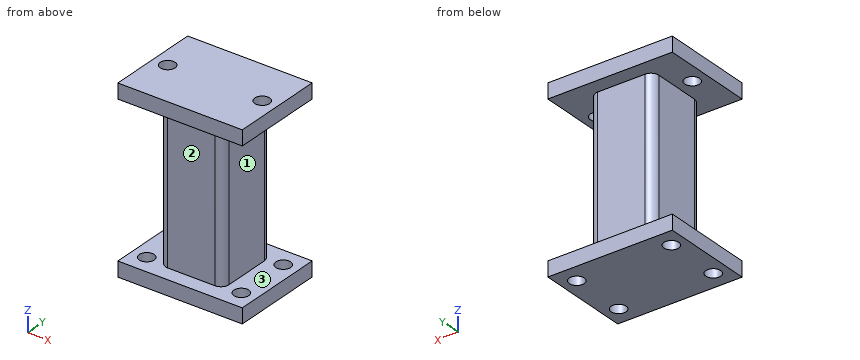
```python
from build123d import *

# Parameters (mm, degrees)
F0_W     = 100
F0_H     = 75
F1_DEPTH = 12
F3_DEPTH = 120.5
F5_W     = 100
F5_H     = 75
F6_DEPTH = 12
F8_D     = 12
F8_DEPTH = 12
F8_TIP   = 3.6051637142
F9_D     = 12
F9_DEPTH = 12
F9_TIP   = 3.6051637142


with BuildPart() as f1:
    # F0 (on Top) → F1 (new body)
    with BuildSketch(Plane.XY):
        Rectangle(F0_W, F0_H)
    extrude(amount=-F1_DEPTH)

    # F2 (on face) → F3 (join)
    with BuildSketch(Plane.XY):
        with BuildLine():
            Line((-19.05, -25.4), (19.05, -25.4))
            ThreePointArc((19.05, -25.4), (23.5401280605, -23.5401280605), (25.4, -19.05))
            Line((25.4, -19.05), (25.4, 19.05))
            ThreePointArc((25.4, 19.05), (23.5401280605, 23.5401280605), (19.05, 25.4))
            Line((19.05, 25.4), (-19.05, 25.4))
            ThreePointArc((-19.05, 25.4), (-23.5401280605, 23.5401280605), (-25.4, 19.05))
            Line((-25.4, 19.05), (-25.4, -19.05))
            ThreePointArc((-25.4, -19.05), (-23.5401280605, -23.5401280605), (-19.05, -25.4))
        make_face()
        with BuildLine():
            Line((-12.7, 19.05), (12.7, 19.05))
            ThreePointArc((12.7, 19.05), (17.1901280605, 17.1901280605), (19.05, 12.7))
            Line((19.05, 12.7), (19.05, -12.7))
            ThreePointArc((19.05, -12.7), (17.1901280605, -17.1901280605), (12.7, -19.05))
            Line((12.7, -19.05), (-12.7, -19.05))
            ThreePointArc((-12.7, -19.05), (-17.1901280605, -17.1901280605), (-19.05, -12.7))
            Line((-19.05, -12.7), (-19.05, 12.7))
            ThreePointArc((-19.05, 12.7), (-17.1901280605, 17.1901280605), (-12.7, 19.05))
        make_face(mode=Mode.SUBTRACT)
    extrude(amount=F3_DEPTH)

    # F5 (on face) → F6 (join)
    with BuildSketch(Plane.XY.offset(120.5)):
        Rectangle(F5_W, F5_H)
        with BuildLine():
            Line((19.05, -25.4), (-19.05, -25.4))
            ThreePointArc((-19.05, -25.4), (-23.5401280605, -23.5401280605), (-25.4, -19.05))
            Line((-25.4, -19.05), (-25.4, 19.05))
            ThreePointArc((-25.4, 19.05), (-23.5401280605, 23.5401280605), (-19.05, 25.4))
            Line((-19.05, 25.4), (19.05, 25.4))
            ThreePointArc((19.05, 25.4), (23.5401280605, 23.5401280605), (25.4, 19.05))
            Line((25.4, 19.05), (25.4, -19.05))
            ThreePointArc((25.4, -19.05), (23.5401280605, -23.5401280605), (19.05, -25.4))
        make_face(mode=Mode.SUBTRACT)
        with BuildLine():
            ThreePointArc((-25.4, -19.05), (-23.5401280605, -23.5401280605), (-19.05, -25.4))
            Line((-19.05, -25.4), (19.05, -25.4))
            ThreePointArc((19.05, -25.4), (23.5401280605, -23.5401280605), (25.4, -19.05))
            Line((25.4, -19.05), (25.4, 19.05))
            ThreePointArc((25.4, 19.05), (23.5401280605, 23.5401280605), (19.05, 25.4))
            Line((19.05, 25.4), (-19.05, 25.4))
            ThreePointArc((-19.05, 25.4), (-23.5401280605, 23.5401280605), (-25.4, 19.05))
            Line((-25.4, 19.05), (-25.4, -19.05))
        make_face()
        with BuildLine():
            Line((-19.05, -12.7), (-19.05, 12.7))
            ThreePointArc((-19.05, 12.7), (-17.1901280605, 17.1901280605), (-12.7, 19.05))
            Line((-12.7, 19.05), (12.7, 19.05))
            ThreePointArc((12.7, 19.05), (17.1901280605, 17.1901280605), (19.05, 12.7))
            Line((19.05, 12.7), (19.05, -12.7))
            ThreePointArc((19.05, -12.7), (17.1901280605, -17.1901280605), (12.7, -19.05))
            Line((12.7, -19.05), (-12.7, -19.05))
            ThreePointArc((-12.7, -19.05), (-17.1901280605, -17.1901280605), (-19.05, -12.7))
        make_face(mode=Mode.SUBTRACT)
        with BuildLine():
            ThreePointArc((-12.7, 19.05), (-17.1901280605, 17.1901280605), (-19.05, 12.7))
            Line((-19.05, 12.7), (-19.05, -12.7))
            ThreePointArc((-19.05, -12.7), (-17.1901280605, -17.1901280605), (-12.7, -19.05))
            Line((-12.7, -19.05), (12.7, -19.05))
            ThreePointArc((12.7, -19.05), (17.1901280605, -17.1901280605), (19.05, -12.7))
            Line((19.05, -12.7), (19.05, 12.7))
            ThreePointArc((19.05, 12.7), (17.1901280605, 17.1901280605), (12.7, 19.05))
            Line((12.7, 19.05), (-12.7, 19.05))
        make_face()
    extrude(amount=F6_DEPTH)

    # F8
    with Locations(Plane.XY.offset(132.5)):
        with Locations((-38, 0), (38, 0)):
            Hole(F8_D / 2, depth=F8_DEPTH)
            with Locations((0, 0, -(F8_DEPTH + F8_TIP / 2))):  # 118° drill point
                Cone(0, F8_D / 2, F8_TIP, mode=Mode.SUBTRACT)

    # F9 (one way)
    with BuildSketch(Plane.XY):
        with Locations((-38, 22.5), (38, 22.5), (38, -22.5), (-38, -22.5)):
            Circle(F9_D / 2)
    extrude(amount=-F9_DEPTH, mode=Mode.SUBTRACT)
    with Locations(Plane.XY):
        with Locations((-38, 22.5), (38, 22.5), (38, -22.5), (-38, -22.5)):
            with Locations((0, 0, -(F9_DEPTH + F9_TIP / 2))):  # 118° drill point
                Cone(0, F9_D / 2, F9_TIP, mode=Mode.SUBTRACT)


solid = f1.part
```
The listing builds one solid part. Answer for the finished solid, in the listing's coordinates (mm). Face numbers are marked on the shaded views. A direction names the side the tool comes from. Coordinates: 2 decimals unless noted, no trailing zeros. Write each loop counter-clockwise with the first axis right and the second up, starting at its lowest first coordinate (ties: lowest second). Pieces come first, ordered by that corner, then holes. Notation, with made-up numbers: (19, 39) -> (29, 39) arc R20 cw to (29, 76) -> close; hole circle Ø7 at (42.25, 77). An arc over 180 degrees is marked (long way). Write each question's results on one line, items separated by ' | '. Start each with the question number.
1) Flat-ended cylindrical pins translate along their axes: pin 1 Ø12 at (x, z) = (13, 107.5) entering from -Y; pin 2 Ø4 at (y, z) = (-11, 48) entering from +X; pin 3 Ø11 at (x, y) = (38, -22.5) entering from -Z. Find the tip coordinate at first contact, or state that the pin passes through.
2) A cutting plane is placed at D-D (z = 37). Determine the outline of the cut face in (x, y), then the cut area to 3 significant figures.
3) A cutting plane is placed at A-A (y = 0). Determine the outline of the cut face in (x, z), then the cut area to 3 significant figures.
4) A cutting plane is placed at B-B (y = -10). Determine the outline of the cut face in (x, z).
5) A tool of negligible diameter and unlimited length cuts with its end or side. For the marked faces 1, 2 and 3, from which of +Z, -Z, +X, -X, +Y, -Y can it reach the whole face along a straight path? Write none if from no direction.
6) Straight lines are drawn through the part: probe 1 along Y at (x, z) = (38, -4); probe 2 along X at (y, z) = (7, 48); probe 3 along Z at (x, y) = (-25, -24). For each, find the intervals that lie inside material, in ascending order.
7) A cutting plane is placed at C-C (x = 38). Determine the outline of the cut face in (y, z), then the cut area to 3 significant figures.
Values follow:
1) pin 1: y = -25.4 | pin 2: x = 25.4 | pin 3: z = 120.5
2) outline: (-25.4, -19.05) arc R6.35 ccw to (-19.05, -25.4) -> (19.05, -25.4) arc R6.35 ccw to (25.4, -19.05) -> (25.4, 19.05) arc R6.35 ccw to (19.05, 25.4) -> (-19.05, 25.4) arc R6.35 ccw to (-25.4, 19.05) -> close; hole (-19.05, -12.7) arc R6.35 ccw to (-12.7, -19.05) -> (12.7, -19.05) arc R6.35 ccw to (19.05, -12.7) -> (19.05, 12.7) arc R6.35 ccw to (12.7, 19.05) -> (-12.7, 19.05) arc R6.35 ccw to (-19.05, 12.7) -> close | area: 1,130 mm²
3) outline: (-50, -12) -> (50, -12) -> (50, 0) -> (25.4, 0) -> (25.4, 120.5) -> (32, 120.5) -> (32, 132.5) -> (-32, 132.5) -> (-32, 120.5) -> (-25.4, 120.5) -> (-25.4, 0) -> (-50, 0) -> close; (-50, 120.5) -> (-44, 120.5) -> (-44, 132.5) -> (-50, 132.5) -> close; (44, 120.5) -> (50, 120.5) -> (50, 132.5) -> (44, 132.5) -> close; hole (-19.05, 0) -> (19.05, 0) -> (19.05, 120.5) -> (-19.05, 120.5) -> close | area: 3,640 mm²
4) outline: (-50, -12) -> (50, -12) -> (50, 0) -> (25.4, 0) -> (25.4, 120.5) -> (50, 120.5) -> (50, 132.5) -> (-50, 132.5) -> (-50, 120.5) -> (-25.4, 120.5) -> (-25.4, 0) -> (-50, 0) -> close; hole (-19.05, 0) -> (19.05, 0) -> (19.05, 120.5) -> (-19.05, 120.5) -> close
5) face 1: +X, +Y, -Y | face 2: +X, -X, -Y | face 3: none
6) probe 1: -37.5 to -28.5, -16.5 to 16.5, 28.5 to 37.5 | probe 2: -25.4 to -19.05, 19.05 to 25.4 | probe 3: -12 to 0, 120.5 to 132.5
7) outline: (-37.5, -12) -> (-28.5, -12) -> (-28.5, 0) -> (-37.5, 0) -> close; (-37.5, 120.5) -> (-6, 120.5) -> (-6, 132.5) -> (-37.5, 132.5) -> close; (-16.5, -12) -> (16.5, -12) -> (16.5, 0) -> (-16.5, 0) -> close; (6, 120.5) -> (37.5, 120.5) -> (37.5, 132.5) -> (6, 132.5) -> close; (28.5, -12) -> (37.5, -12) -> (37.5, 0) -> (28.5, 0) -> close | area: 1,370 mm²
